Build history of the part. All positions in model axes, mm. A direction names the side the tool comes from. Round coordinates to 2 decimals unless told otherwise and drop trailing zeros. Write each loop counter-clockwise with the first axis right and the second up, starting at its lowest first coordinate (ties: lowest second). Pieces come first, ordered by that corner, then holes. Notation, with made-up numbers: M 52.25,-18.5 L 81.25,-18.5 A18 ccw 81.25,-13.5 Z; hole C 4,23.5 d4. An arc over 180 degrees is marked long. Write item = value, one per line. Start each with the question number.
Q1. Probe L1, parallel to Y at x = 3, z = 4; L2, parallel to Y at x = 4.75, z = 8. List the from-to ranges inside material, lowest first.
Q2. Drop flat-ended pins along their axis: P1, Ø3, axis at y = 2.5, z = 5.5, coming from the -X side; P2, Ø4, axis at x = 2, y = -4, coming from the +Z side; P3, Ø1.5, axis at x = 2, z = 6.5, coming from the +Y side; P4, Ø3.5, axis at x = 3, y = -8, coming from the -Z side. Give the stop position or say it passes through.
Q3. Tool access for faces 5 (the cylindrical face through (0.301, 5.715, 5.056)), 6 (the flat face through (6, 3, 5)), 7 (the cylindrical face through (5.715, 5.699, 5.056)), 8 (the cylindrical face through (5.699, 0.285, 5.056)), 9 (the cylindrical face through (0.285, 0.301, 5.056)): list every direction of +Z, -Z, +X, -X, +Y, -Y with a clear straight run to the whole face (end or side of a thin tool).
Q4. Band-saw the part on A-A on z = 8.75. Write the cut outline in (x, y).
Q5. Pull direction Y, two halves, no side cores. Call faces 1 (the flat face through (3, -5, 0)), 2 (the flat face through (3, 0, 5)), 3 (the cylindrical face through (3.85, -6.89, -1.01)), 4 (the conical face through (2.87, 3.17, 1.39)): released by +Y, released by -Y, zero draft, split by the parting line, or undercut.
Autodesk Inventor part; units mm, degrees
ref_plane "YZ Plane" through (0, 0, 0) normal (1, 0, 0) x (0, 1, 0)
ref_plane "XZ Plane" through (0, 0, 0) normal (0, 1, 0) x (-1, 0, 0)
ref_plane "XY Plane" through (0, 0, 0) normal (0, 0, 1) x (1, 0, 0)
sketch "Sketch1" plane through (0, 0, 0) normal (0, 0, 1) x (1, 0, 0)
  line L0 (0, 0) -> (6, 0)
  line L1 (6, 0) -> (6, 6)
  line L2 (6, 6) -> (0, 6)
  line L3 (0, 6) -> (0, 0)
  dimension "d0" = 6
  dimension "d1" = 6
extrude "Extrusion1" add sketch "Sketch1" along normal blind 10
sketch "Sketch8" plane through (0, 0, 0) normal (0, 0, -1) x (-1, 0, 0)
  line L0 (0, 0) -> (-6, 0)
  line L1 (0, 6) -> (0, 0)
  line L2 (-6, 6) -> (0, 6)
  line L3 (-6, 0) -> (-6, 6)
  line L4 (-8, 8) -> (2, 8)
  line L5 (2, 8) -> (2, -11)
  line L6 (2, -11) -> (-8, -11)
  line L7 (-8, -11) -> (-8, 8)
  dimension "d46" = 2
  dimension "d47" = 2
  dimension "d48" = 2
  dimension "d49" = 11
extrude "Extrusion4" add sketch "Sketch8" along normal blind 2 contours L0 L3 L2 L1 | L4 L5 L6 L7
sketch "Sketch9" plane through (0, 0, 10) normal (0, 0, 1) x (1, 0, 0)
  line L0 (0, 6) -> (6, 0) construction
  line L1 (0, 0) -> (6, 6) construction
  point P0 (3, 3)
hole "Hole5" at (3, 3, 10) direction (0, 0, -1) diameter 2.459 depth 8 tip angle 118
sketch "Sketch10" plane through (0, 0, 0) normal (0, 0, 1) x (1, 0, 0)
  line L0 (8, 8) -> (-2, 8)
  line L1 (-2, -11) -> (8, -11)
  line L2 (3, -11) -> (3, 8) construction
  point P0 (3, -8)
  dimension "d59" = 3
hole "Hole6" at (3, -8, 0) direction (0, 0, -1) diameter 2.8 end through all
fillet "Fillet4" radius 5 2 edges at (8, -11, -1) (-2, -11, -1)
fillet "Fillet5" radius 1 8 edges at (0, 0, 5) (0, 3, 10) (0, 6, 5) (3, 6, 10) (6, 6, 5) (6, 3, 10) (6, 0, 5) (3, 0, 10)
fillet "Fillet6" radius 1 8 edges at (3, 6, 0) (0.2929, 5.7071, 0) (0, 3, 0) (0.2929, 0.2929, 0) (3, 0, 0) (5.7071, 0.2929, 0) (6, 3, 0) (5.7071, 5.7071, 0)
fillet "Fillet8" radius 0.999 4 edges at (8, 8, -1) (-2, 8, -1) (3, 8, 0) (3, 8, -2)
fillet "Fillet9" radius 0.999 10 edges at (7.7074, 7.7074, -0.2926) (-0.5356, -9.5356, 0) (-2, 0.5005, 0) (-1.7074, 7.7074, -0.2926) (8, 0.5005, 0) (-0.5356, -9.5356, -2) (-2, 0.5005, -2) (-1.7074, 7.7074, -1.7074) (7.7074, 7.7074, -1.7074) (8, 0.5005, -2)
properties part number "termination_lv_conductor" material "Copper, Cast"
Conclusion:
q1.L1 = 0 to 1.77, 4.23 to 6
q1.L2 = 0 to 6
q2.P1 = 0
q2.P2 = 0
q2.P3 = 6
q2.P4 = -2
q3.face_5 = +Z, -X, +Y
q3.face_6 = +Z, +X, +Y, -Y
q3.face_7 = +Z, +X, +Y
q3.face_8 = +Z, +X, -Y
q3.face_9 = +Z, -X, -Y
q4.outline = M 0,1 A1 ccw 1,0 L 5,0 A1 ccw 6,1 L 6,5 A1 ccw 5,6 L 1,6 A1 ccw 0,5 Z; hole C 3,3 d2.46
q5.face_1 = zero draft
q5.face_2 = released by -Y
q5.face_3 = undercut
q5.face_4 = undercut
